Read the model definition and answer for the solid it produces. Units are mm, in the model's axes. Face numbers are marked on the shaded views. Give positions to 0.01 mm unless a question says otherwise; leave off trailing zeros. Loops run counter-clockwise (first coordinate to the right, second up) from the corner with the lowest first, then second, coordinate; pieces in that order, holes last. Notation, with made-up numbers: (61, 21) - (88, 21) arc R20 ccw to (88, 31) - close; hole circle Ø8 at (55.25, 3.25). An arc over 180 degrees is marked (long way). Write item = value, one per line.
```python
from build123d import *

# Parameters (mm, degrees)
BOSS_EXTRUDE2_DEPTH = 0.5
SKETCH3_R           = 1
CUT_EXTRUDE2_DEPTH  = 1.5000001


with BuildPart() as part:
    # Sketch1 → Boss-Extrude2 (new body)
    with BuildSketch(Plane(origin=(0, 0, 0), x_dir=(1, 0, 0), z_dir=(0, 1, 0))):
        with BuildLine():
            Line((64.487313154, 0.25), (4, 0.25))
            ThreePointArc((4, 0.25), (0, 4.007804885), (-4, 0.25))
            Line((-4, 0.25), (-12.67773598, 0.606260641))
            add(Edge.make_bspline(
                [(-12.67773598, -0.606260641), (-13.533789945, 0), (-12.67773598, 0.606260641)],
                knots=[0, 0, 0, 1, 1, 1], degree=2))
            Line((-12.67773598, -0.606260641), (-4, -0.25))
            ThreePointArc((-4, -0.25), (0, -4.007804885), (4, -0.25))
            Line((4, -0.25), (64.487313154, -0.25))
            Line((64.487313154, -0.25), (64.487313154, 0.25))
        make_face()
    extrude(amount=BOSS_EXTRUDE2_DEPTH)

    # Sketch3 → Cut-Extrude2 (cut, through all)
    with BuildSketch(Plane(origin=(0, 0.5, 0), x_dir=(1, 0, 0), z_dir=(0, 1, 0))):
        Circle(SKETCH3_R)
    extrude(amount=-CUT_EXTRUDE2_DEPTH, mode=Mode.SUBTRACT)


solid = part.part
```
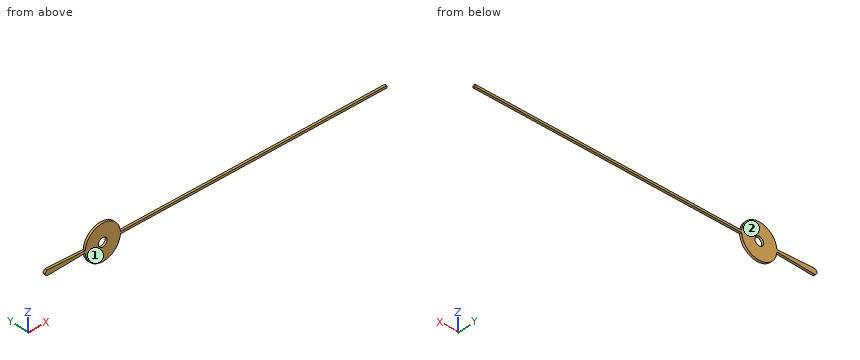
1) This flat-tipped pin is pushed along its axis until it touches: P1, Ø2, axis at x = 23.5, z = -3, coming from the +Y side. Where does it stop, or does it pass through?
Output:
P1 = through
2) Find the intervals of material crossed by probe 1 along X at (y, z) = (0.3, 0); probe 2 along Z at (x, y) = (30.5, 0.4); probe 3 along X at (y, z) = (0.45, 0.75), in increasing order.
Output:
probe_1 = -13.11 to -1, 1 to 64.49
probe_2 = -0.25 to 0.25
probe_3 = -3.94 to -0.66, 0.66 to 3.94
3) The mould has two halves that part along Y. Classify the marked faces 1 and 2: pulls with the +Y half, pulls with the -Y half, needs draft (parallel to the pull), parting line crosses it, or undercut.
Output:
face_1 = pulls with the -Y half
face_2 = pulls with the +Y half
4) A cutting plane is placed at C-C on x = 45. Determine the outline of the cut face in (y, z), then the cut area to 3 significant figures.
Output:
outline = (0, -0.25) - (0.5, -0.25) - (0.5, 0.25) - (0, 0.25) - close
area = 0.250 mm²
5) A cutting plane is placed at A-A on x = 0. Determine the outline of the cut face in (y, z).
Output:
outline = (0, -4.01) - (0.5, -4.01) - (0.5, -1) - (0, -1) - close; (0, 1) - (0.5, 1) - (0.5, 4.01) - (0, 4.01) - close
6) A cutting plane is placed at B-B on z = -2.75. Determine the outline of the cut face in (x, y), then the cut area to 3 significant figures.
Output:
outline = (-2.92, 0) - (2.92, 0) - (2.92, 0.5) - (-2.92, 0.5) - close
area = 2.92 mm²
